Check sheet for the modelled part. Datum: model origin and axes. Units: mm. A direction names the side the tool comes from. Round coordinates to 2 decimals unless told otherwise and drop trailing zeros. Order: outer loops, then holes, each group sorted by start corner. A loop starts at its lowest first (then second) coordinate and runs counter-clockwise, first axis right, second up. Notation, with made-up numbers: (75, 6.5) -> (112, 6.5) arc R26 ccw to (112, 25.5) -> close; hole circle Ø10 at (80, 78). An arc over 180 degrees is marked (long way). Answer in a Markdown table with one row per item.
from build123d import *

# Parameters (mm, degrees)
F0_R     = 3.9751
F0_R_2   = 3.96875
F1_DEPTH = 3.175
F3_DEPTH = 25.4


with BuildPart() as f1:
    # F0 (on Top) → F1 (new body)
    with BuildSketch(Plane.XY):
        Polygon((-102.986208, 11.167409), (-102.986208, -102.693632), (100.37496, -102.693632), (100.366036, 11.175378), align=None)
        with Locations((-82.336008, -83.478532)):
            Circle(F0_R, mode=Mode.SUBTRACT)
        with Locations((79.715992, -83.478532)):
            Circle(F0_R, mode=Mode.SUBTRACT)
        with Locations((-82.336008, -5.500532)):
            Circle(F0_R_2, mode=Mode.SUBTRACT)
        with Locations((79.715992, -5.500532)):
            Circle(F0_R, mode=Mode.SUBTRACT)
    extrude(amount=F1_DEPTH)

    # F2 (on face) → F3 (join)
    with BuildSketch(Plane(origin=(0, 0, 0), x_dir=(1, 0, 0), z_dir=(0, 0, -1))):
        Polygon((100.37496, 102.693632), (-102.986208, 102.693632), (-102.986208, -11.167409), (100.366036, -11.175378), align=None)
        Polygon((-99.811208, -7.992534), (-99.811208, 99.518632), (97.199711, 99.518632), (97.191285, -8.000253), align=None, mode=Mode.SUBTRACT)
    extrude(amount=F3_DEPTH)


solid = f1.part
Item 1: Cross-section at B-B (y = 4). Record the boundary of the cut face in (x, z) (3 decimals).
Result sheet:
| item | result |
|---|---|
| outline | (-102.986, -25.4) -> (-99.811, -25.4) -> (-99.811, 0) -> (97.192, 0) -> (97.192, -25.4) -> (100.367, -25.4) -> (100.367, 3.175) -> (-102.986, 3.175) -> close |
Item 2: Scan lines: line 1 (Y direction, x = -15, z = -10.25); line 2 (X direction, y = 0, z = -3.25); line 3 (X direction, y = -81.5, z = 1.75). Record each from-to range of solid material in increasing order. Write a range as [from, to].
Result sheet:
| item | result |
|---|---|
| line 1 | y = [-102.69, -99.52], [8, 11.17] |
| line 2 | x = [-102.99, -99.81], [97.19, 100.37] |
| line 3 | x = [-102.99, -85.78], [-78.89, 76.27], [83.16, 100.37] |
Item 3: Cross-section at C-C (x = -41). Record the boundary of the cut face in (y, z) (3 decimals).
Result sheet:
| item | result |
|---|---|
| outline | (-102.694, -25.4) -> (-99.519, -25.4) -> (-99.519, 0) -> (7.995, 0) -> (7.995, -25.4) -> (11.17, -25.4) -> (11.17, 3.175) -> (-102.694, 3.175) -> close |
Item 4: Set-up check for faces 1 (the cylindrical face through (-82.853, -79.537, 1.565)), 2 (the flat face through (-3, -99.519, -13)): record each of +Z, -Z, +X, -X, +Y, -Y from which the full face is reachable in a straight line by a thin tool's end or side.
Result sheet:
| item | result |
|---|---|
| face 1 | +Z, -Z |
| face 2 | -Z |
Item 5: Cross-section at A-A (z = -12). Record the boundary of the cut face in (x, y), and give its area (3 significant figures).
Result sheet:
| item | result |
|---|---|
| outline | (-102.99, -102.69) -> (100.37, -102.69) -> (100.37, 11.18) -> (-102.99, 11.17) -> close; hole (-99.81, -99.52) -> (97.2, -99.52) -> (97.19, 8) -> (-99.81, 7.99) -> close |
| area | 1,970 mm^2 |
Item 6: Depth check by flat-ended pin: P1, Ø12.5, axis at x = -82.34, y = -83.48, coming from the +Z side (3 decimals); P2, Ø8.5, axis at y = -56, z = -7, coming from the +X side; P3, Ø4, axis at x = -23, z = -4.5, coming from the +Y side; P4, Ø1.5, axis at x = -42.5, y = -22, coming from the -Z side. Enter the tip coordinate at first touch or a pass-through.
Result sheet:
| item | result |
|---|---|
| P1 | stops at z = 3.175 |
| P2 | stops at x = 100.37 |
| P3 | stops at y = 11.17 |
| P4 | stops at z = 0 |
